Can you work these out from the drawing? Everything is in mm from the part's minimum corner. A direction names the side the tool comes from. Coordinates: 2 decimals unless noted, no trailing zeros. Write each loop counter-clockwise with the first axis right and the second up, starting at its lowest first coordinate (ties: lowest second). Pieces come first, ordered by that corner, then holes. Notation, with made-up numbers: M -31,88 L 28,88 A25 cw 28,121 Z; hole C -17,13.25 d7. An arc over 180 degrees is marked long. Write item = value, one per line.
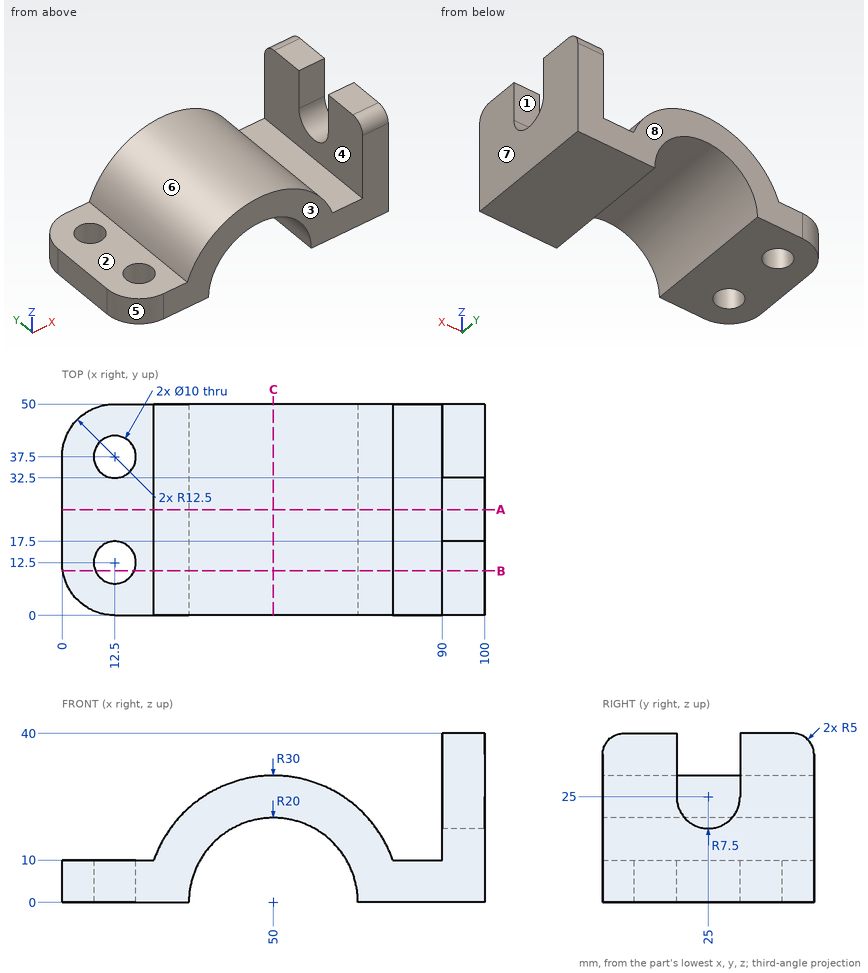
Item 1: Imagine slicing it at C-C (x = 50). Write out the boundary of the cut face in (y, z).
Numbers:
outline = M 0,20 L 50,20 L 50,30 L 0,30 Z
Item 2: If we mould it in two halves opening along X, with no side actions, what happens to the marked faces 5, 6, 7 and 8? For each: pulls with the +X half, pulls with the -X half, needs draft (parallel to the pull), parting line crosses it, or undercut.
Numbers:
face_5 = pulls with the -X half
face_6 = undercut
face_7 = pulls with the +X half
face_8 = needs draft
Item 3: Imagine slicing it at B-B (y = 10.5). Write out the boundary of the cut face in (x, z).
Numbers:
outline = M 0.16,0 L 7.92,0 L 7.92,10 L 0.16,10 Z; M 17.08,0 L 30,0 A20 cw 70,0 L 100,0 L 100,40 L 90,40 L 90,10 L 78.28,10 A30 ccw 21.72,10 L 17.08,10 Z
Item 4: For the marked faces 1, 2, 3 and 4, which set-ups out of +Z, -Z, +X, -X, +Y, -Y let a thin tool reach every point of the face, with its end or its side?
Numbers:
face_1 = +Z, +X
face_2 = +Z, -X, +Y, -Y
face_3 = +Z, -Z, +X, -X, -Y
face_4 = +Z, +Y, -Y
Item 5: If I drill on line 1 along Y through (x, z) = (12.5, 8.25); line 2 along Y through (x, z) = (94, 25); line 3 along X through (y, z) = (37, 7) (3 decimals), over which ranges is the centre line in solid material (lowest first)?
Numbers:
line_1 = 0 to 7.5, 17.5 to 32.5, 42.5 to 50
line_2 = 0 to 17.5, 32.5 to 50
line_3 = 0 to 7.525, 17.475 to 31.265, 68.735 to 100
Item 6: Imagine slicing it at A-A (y = 25). Write out the boundary of the cut face in (x, z).
Numbers:
outline = M 0,0 L 30,0 A20 cw 70,0 L 100,0 L 100,17.5 L 90,17.5 L 90,10 L 78.28,10 A30 ccw 21.72,10 L 0,10 Z
Item 7: I'm going to push flat-ended pins straight in: P1, Ø10, axis at x = 75, z = 12.5, coming from the -Y side; P2, Ø6.5, axis at x = 6.5, y = 13, coming from the +Z side; P3, Ø10, axis at x = 18, y = 16, coming from the +Z side; P4, Ø1.5, axis at y = 41, z = 6, coming from the -X side. Where does each tip first touch, or does it pass through?
Numbers:
P1 = 0
P2 = 10
P3 = 13.08
P4 = 0.31
